Can you work these out from the drawing? Everything is in mm from the part's minimum corner. A direction names the side the tool comes from. Round coordinates to 2 decimals unless told otherwise and drop trailing zeros. Write each loop counter-clockwise with the first axis right and the second up, starting at its lowest first coordinate (ties: lowest second). Pieces come first, ordered by that corner, then holes. Notation, with made-up numbers: M -19,0 L 37,0 A22 ccw 37,26 Z; hole C -23.5,79.25 d1. An arc over 180 degrees is marked long. Answer in a Markdown table with one row per item. Add a question column.
(1) Suppose I cut it at A-A, the plane y = 17.5. Write out the boundary of the cut face in (x, z).
(2) For the marked faces 1 and 2, which set-ups out of +Z, -Z, +X, -X, +Y, -Y let a thin tool reach every point of the face, with its end or its side?
(3) Suppose I cut it at C-C, the plane z = 10. Write out the boundary of the cut face in (x, y), then the cut area to 3 significant figures.
(4) I'm going to push flat-ended pins straight in: pin 1 (10 mm diameter, centred on x = 11.5, z = 15, fed in from -Y); pin 2 (5 mm diameter, centred on y = 20.5, z = 7.5, fed in from +X); pin 3 (1 mm diameter, centred on y = 5, z = 4.5, fed in from +X); pin 4 (3 mm diameter, centred on x = 19, y = 18, fed in from +Z). Where does each tip first touch, or does it pass through?
(5) Suppose I cut it at D-D, the plane y = 3.5. Write out the boundary of the cut face in (x, z), then the cut area to 3 significant figures.
(6) If I drill on probe 1 along Z at (x, y) = (30.5, 14.5); probe 2 along Y at (x, z) = (17.5, 11); probe 3 along Y at (x, z) = (14, 11), over which ranges is the centre line in solid material (lowest first)?
(7) Suppose I cut it at B-B, the plane x = 17.5. Write out the boundary of the cut face in (y, z), then the cut area to 3 significant figures.
(8) If we mould it in two halves opening along Z, with no side actions, what happens to the marked faces 3, 4 and 5? For each: released by +Z, released by -Z, zero draft, split by the parting line, or undercut.
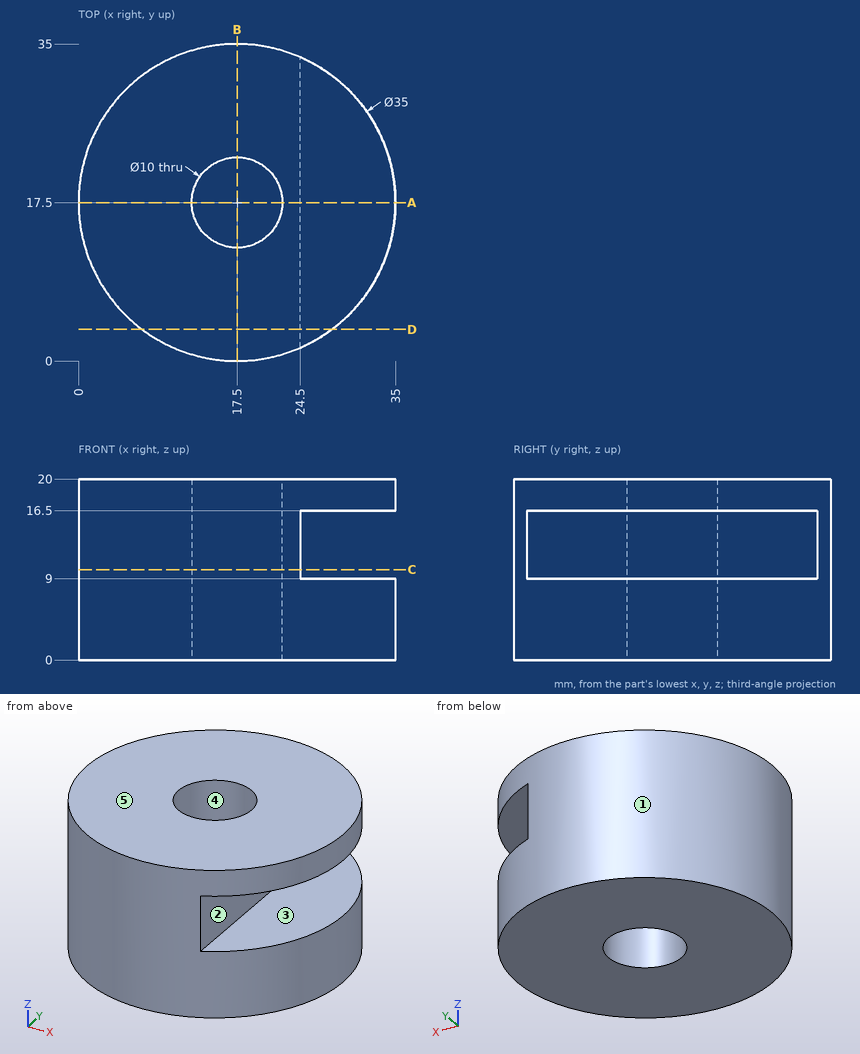
Calculated:
| question | item | result |
|---|---|---|
| 1 | outline | M 0,0 L 12.5,0 L 12.5,20 L 0,20 Z; M 22.5,0 L 35,0 L 35,9 L 24.5,9 L 24.5,16.5 L 35,16.5 L 35,20 L 22.5,20 Z |
| 2 | face 1 | +Z, -Z |
| 2 | face 2 | +X, +Y, -Y |
| 3 | outline | M 24.5,1.46 L 24.5,33.54 A17.5 ccw long Z; hole C 17.5,17.5 d10 |
| 3 | area | 641 mm² |
| 4 | pin 1 | y = 0.03 |
| 4 | pin 2 | x = 34.99 |
| 4 | pin 3 | x = 30.24 |
| 4 | pin 4 | through |
| 5 | outline | M 7,0 L 28,0 L 28,9 L 24.5,9 L 24.5,16.5 L 28,16.5 L 28,20 L 7,20 Z |
| 5 | area | 394 mm² |
| 6 | probe 1 | 0 to 9, 16.5 to 20 |
| 6 | probe 2 | 0 to 12.5, 22.5 to 35 |
| 6 | probe 3 | 0.35 to 13.93, 21.07 to 34.65 |
| 7 | outline | M 0,0 L 12.5,0 L 12.5,20 L 0,20 Z; M 22.5,0 L 35,0 L 35,20 L 22.5,20 Z |
| 7 | area | 500 mm² |
| 8 | face 3 | undercut |
| 8 | face 4 | zero draft |
| 8 | face 5 | released by +Z |
